Input: dimensioned drawing with shaded views. Units: mm. Origin: part minimum x, y, z. Give positions to 0.01 mm unless a question says otherwise; leave off trailing zeros. Order: outer loops, then holes, each group sorted by start corner. A loop starts at its lowest first (then second) coordinate and runs counter-clockwise, first axis right, second up. Notation, with made-up numbers: (31, -38) - (53, -38) arc R27 cw to (53, -4) - close; hole circle Ø2 at (72, -14). An arc over 180 degrees is marked (long way). Answer as CSV lines item,"result".
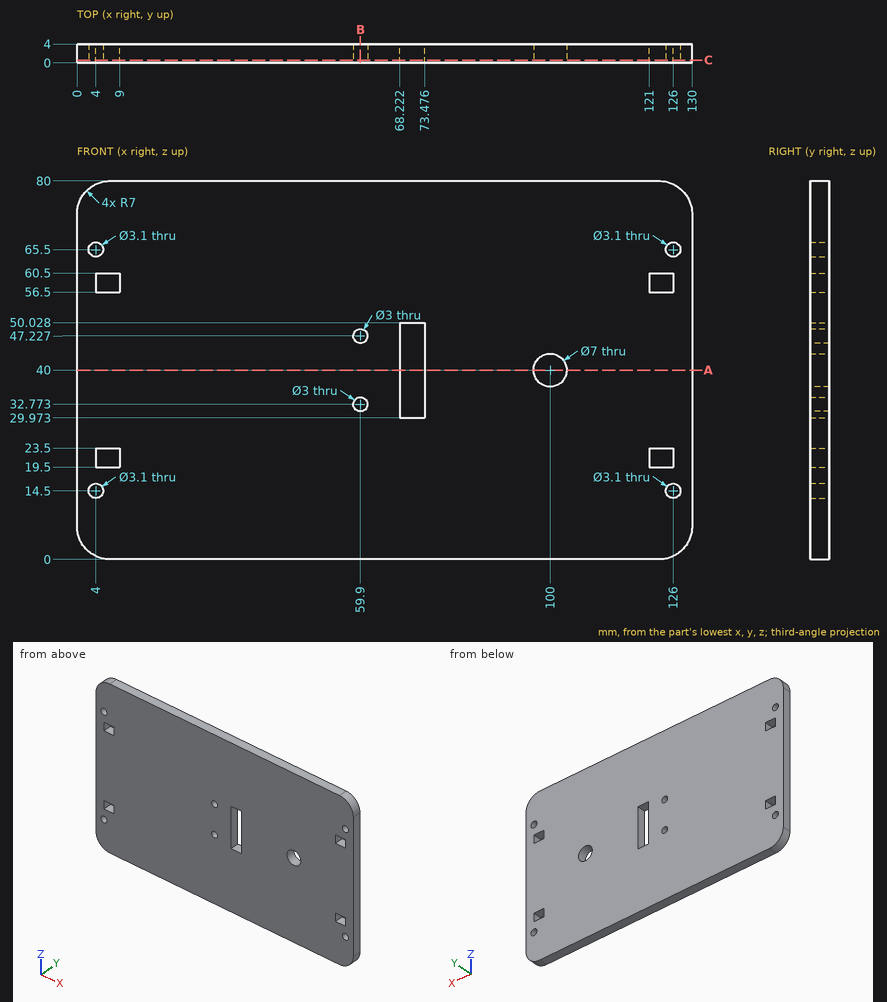
(1) Ray query, line 1 (X direction, y = 0.9, z = 32.5) (1 decimal); line 2 (X direction, y = 1, z = 65.5); line 3 (X direction, y = 0.9, z = 30.5) (1 decimal). Return the intervals inside material, ascending. Write a range as from..to.
Completed:
line 1,"0..58.4, 61.4..68.2, 73.5..130"
line 2,"0..2.45, 5.55..124.45, 127.55..130"
line 3,"0..68.2, 73.5..130"
(2) Cut plane B-B (x = 59.9). Return loops of the section in (y, z).
Completed:
outline,"(0, 0) - (4, 0) - (4, 31.27) - (0, 31.27) - close; (0, 34.27) - (4, 34.27) - (4, 45.73) - (0, 45.73) - close; (0, 48.73) - (4, 48.73) - (4, 80) - (0, 80) - close"
(3) Cut plane A-A (z = 40). Return loops of the section in (x, y) (1 decimal), then the cut area to 3 significant figures.
Completed:
outline,"(0, 0) - (68.2, 0) - (68.2, 4) - (0, 4) - close; (73.5, 0) - (96.5, 0) - (96.5, 4) - (73.5, 4) - close; (103.5, 0) - (130, 0) - (130, 4) - (103.5, 4) - close"
area,"471 mm²"
(4) Contact query for flat-ended pins moving along their axis: pin 1 (2 mm diameter, centred on x = 90, y = 2.5, fed in from -Z); pin 2 (1.2 mm diameter, centred on x = 6, y = 2.5, fed in from +Z). Output: stop coordinate, or through.
Completed:
pin 1,"z = 0"
pin 2,"z = 79.99"
(5) Cut plane C-C (y = 0.6). Give the number of separate pieces and of enclosed holes in the cut face, then the cut area to 3 significant figures.
Completed:
separate pieces,"1"
enclosed holes,"12"
area,"10,100 mm²"
